from build123d import *

# Parameters (mm, degrees)
F1_DEPTH = 9.525
F2_DEPTH = 6.35


with BuildPart() as f1:
    # F0 (on Top) → F1 (new body)
    with BuildSketch(Plane.XY):
        with BuildLine():
            Line((109.0079811876, -106.5036151378), (78.4525489868, -64.5581718877))
            ThreePointArc((78.4525489868, -64.5581718877), (69.69265157, -73.9289815778), (59.8218109514, -82.1213183923))
            Line((59.8218109514, -82.1213183923), (64.495389932, -88.5370463917))
            ThreePointArc((64.495389932, -88.5370463917), (69.459011135, -88.1417123974), (72.0620373203, -92.3864831914))
            ThreePointArc((72.0620373203, -92.3864831914), (71.5443081143, -94.5459570061), (70.1036847087, -96.235919991))
            Line((70.1036847087, -96.235919991), (79.4508426698, -109.0673759898))
            ThreePointArc((79.4508426698, -109.0673759898), (84.4144638729, -108.6720419955), (87.0174900582, -112.9168127895))
            ThreePointArc((87.0174900582, -112.9168127895), (86.4997608522, -115.0762866042), (85.0591374465, -116.7662495891))
            Line((85.0591374465, -116.7662495891), (89.7327164271, -123.1819775885))
            ThreePointArc((89.7327164271, -123.1819775885), (99.7196478413, -115.2464829589), (109.0079811876, -106.5036151378))
        make_face()
        with BuildLine():
            ThreePointArc((59.8218109514, -82.1213183923), (48.9973735962, -89.0045919078), (37.3918882403, -94.469077977))
            Line((37.3918882403, -94.469077977), (67.9473205258, -136.4145213434))
            ThreePointArc((67.9473205258, -136.4145213434), (79.1171509025, -130.254506383), (89.7327164271, -123.1819775885))
            Line((89.7327164271, -123.1819775885), (85.0591374465, -116.7662495891))
            ThreePointArc((85.0591374465, -116.7662495891), (78.4055532585, -115.7209601778), (79.4508426698, -109.0673759898))
            Line((79.4508426698, -109.0673759898), (70.1036847087, -96.235919991))
            ThreePointArc((70.1036847087, -96.235919991), (63.4501005207, -95.1906305797), (64.495389932, -88.5370463917))
            Line((64.495389932, -88.5370463917), (59.8218109514, -82.1213183923))
        make_face()
        with BuildLine():
            Line((67.9473205258, -136.4145213434), (37.3918882403, -94.469077977))
            ThreePointArc((37.3918882403, -94.469077977), (0.3678617573, -101.5993340418), (-36.7068265087, -94.7373679582))
            Line((-36.7068265087, -94.7373679582), (-55.0602397631, -142.1060519374))
            ThreePointArc((-55.0602397631, -142.1060519374), (7.0439756368, -152.2371255878), (67.9473205258, -136.4145213434))
        make_face()
    extrude(amount=-F1_DEPTH)

    # F0 (on Top) → F2 (cut)
    with BuildSketch(Plane.XY):
        with BuildLine():
            ThreePointArc((59.8218109514, -82.1213183923), (48.9973735962, -89.0045919078), (37.3918882403, -94.469077977))
            Line((37.3918882403, -94.469077977), (67.9473205258, -136.4145213434))
            ThreePointArc((67.9473205258, -136.4145213434), (79.1171509025, -130.254506383), (89.7327164271, -123.1819775885))
            Line((89.7327164271, -123.1819775885), (85.0591374465, -116.7662495891))
            ThreePointArc((85.0591374465, -116.7662495891), (78.4055532585, -115.7209601778), (79.4508426698, -109.0673759898))
            Line((79.4508426698, -109.0673759898), (70.1036847087, -96.235919991))
            ThreePointArc((70.1036847087, -96.235919991), (63.4501005207, -95.1906305797), (64.495389932, -88.5370463917))
            Line((64.495389932, -88.5370463917), (59.8218109514, -82.1213183923))
        make_face()
        with BuildLine():
            Line((109.0079811876, -106.5036151378), (78.4525489868, -64.5581718877))
            ThreePointArc((78.4525489868, -64.5581718877), (69.69265157, -73.9289815778), (59.8218109514, -82.1213183923))
            Line((59.8218109514, -82.1213183923), (64.495389932, -88.5370463917))
            ThreePointArc((64.495389932, -88.5370463917), (69.459011135, -88.1417123974), (72.0620373203, -92.3864831914))
            ThreePointArc((72.0620373203, -92.3864831914), (71.5443081143, -94.5459570061), (70.1036847087, -96.235919991))
            Line((70.1036847087, -96.235919991), (79.4508426698, -109.0673759898))
            ThreePointArc((79.4508426698, -109.0673759898), (84.4144638729, -108.6720419955), (87.0174900582, -112.9168127895))
            ThreePointArc((87.0174900582, -112.9168127895), (86.4997608522, -115.0762866042), (85.0591374465, -116.7662495891))
            Line((85.0591374465, -116.7662495891), (89.7327164271, -123.1819775885))
            ThreePointArc((89.7327164271, -123.1819775885), (99.7196478413, -115.2464829589), (109.0079811876, -106.5036151378))
        make_face()
    extrude(amount=-F2_DEPTH, mode=Mode.SUBTRACT)


solid = f1.part
Model file for the job. Use its own axes, mm. A direction names the side the tool comes from. Give positions to 0.01 mm unless a question says otherwise; leave off trailing zeros. Write each loop counter-clockwise with the first axis right and the second up, starting at its lowest first coordinate (ties: lowest second). Pieces come first, ordered by that corner, then holes. Notation, with made-up numbers: (-30.5, -38) -> (-16.5, -38) arc R20 ccw to (-16.5, 1) -> close; hole circle Ø3 at (36, 71). An arc over 180 degrees is marked (long way). Write item = value, one per line.
(1) Slice it at C-C, the plane x = 50.5. Give the cut face in (y, z) (3 decimals), then the cut area to 3 significant figures.
Determined:
outline = (-143.79, -9.525) -> (-88.161, -9.525) -> (-88.161, -6.35) -> (-112.463, -6.35) -> (-112.463, 0) -> (-143.79, 0) -> close
area = 376 mm2
(2) Slice it at B-B, the plane x = 31.5. Give the cut face in (y, z) (3 decimals).
Determined:
outline = (-149.109, -9.525) -> (-96.594, -9.525) -> (-96.594, 0) -> (-149.109, 0) -> close
(3) Probe line 1 along Z through (x, y) = (92.5, -90.5) (3 decimals); line 2 along X through (y, z) = (-92, -7); line 3 along X through (y, z) = (-92.5, -8.75). List the from-to ranges inside material, lowest first.
Determined:
line_1 = -9.525 to -6.35
line_2 = 43.11 to 62.55, 72.05 to 98.44
line_3 = 42.03 to 62.54, 72.06 to 98.81
(4) Slice it at A-A, the plane z = -2.75. Give the cut face in (x, y), then the cut area to 3 significant figures.
Determined:
outline = (-55.06, -142.11) arc R152.4 ccw to (67.95, -136.41) -> (37.39, -94.47) arc R101.6 cw to (-36.71, -94.74) -> close
area = 5,150 mm2
(5) Tool access for faces 1 (the face through (93.94, -85.82, -7.92)), 2 (the face through (52.456, -115.148, -3.131)): list every direction of +Z, -Z, +X, -X, +Y, -Y with a clear straight run to the whole face (end or side of a thin tool).
Determined:
face_1 = +Z, -Z, +X, +Y
face_2 = +Z, +X, +Y
(6) Flat gauge pins, fed straight in: P1, Ø3, axis at x = 21.5, z = -8.5, coming from the -Y side; P2, Ø3, axis at x = 34, z = -8.5, coming from the -Y side; P3, Ø1.5, axis at y = -111.5, z = -2.5, coming from the -X side. Where does each tip first touch, or does it go through?
Determined:
P1 = -151.08
P2 = -148.89
P3 = -43.49
